```python
from build123d import *

# Parameters (mm, degrees)
SKETCH1_W           = 82.55
SKETCH1_H           = 44.45
BOSS_EXTRUDE1_DEPTH = 6.35
SKETCH2_W           = 5.588
SKETCH2_H           = 18.288
BOSS_EXTRUDE2_DEPTH = 6.35
SKETCH5_W           = 18.288
SKETCH5_H           = 5.588
BOSS_EXTRUDE3_DEPTH = 6.35
SKETCH3_W           = 5.588
SKETCH3_H           = 18.288
CUT_EXTRUDE1_DEPTH  = 97.739994025
SKETCH6_R           = 1.524
CUT_EXTRUDE2_DEPTH  = 97.739994025


with BuildPart() as part:
    # Sketch1 → Boss-Extrude1 (new body)
    with BuildSketch(Plane.XY):
        with Locations((41.275, 22.225)):
            Rectangle(SKETCH1_W, SKETCH1_H)
    extrude(amount=BOSS_EXTRUDE1_DEPTH)

    # Sketch2 → Boss-Extrude2 (add)
    with BuildSketch(Plane.XY.offset(6.35)):
        with Locations((-2.794, 22.225)):
            Rectangle(SKETCH2_W, SKETCH2_H)
    extrude(amount=-BOSS_EXTRUDE2_DEPTH)

    # Sketch5 → Boss-Extrude3 (add)
    with BuildSketch(Plane.XY.offset(6.35)):
        with Locations((38.481, 47.244)):
            Rectangle(SKETCH5_W, SKETCH5_H)
        with Locations((38.481, -2.794)):
            Rectangle(SKETCH5_W, SKETCH5_H)
    extrude(amount=-BOSS_EXTRUDE3_DEPTH)

    # Sketch3 → Cut-Extrude1 (cut, through all)
    with BuildSketch(Plane.XY.offset(6.35)):
        with Locations((79.756, 22.225)):
            Rectangle(SKETCH3_W, SKETCH3_H)
    extrude(amount=-CUT_EXTRUDE1_DEPTH, mode=Mode.SUBTRACT)

    # Sketch6 → Cut-Extrude2 (cut, through all)
    with BuildSketch(Plane.XY.offset(6.35)):
        with Locations((-2.794, 22.225)):
            Circle(SKETCH6_R)
        with Locations((38.481, -2.794)):
            Circle(SKETCH6_R)
        Polygon((67.437, 23.8125), (70.612, 23.8125), (70.612, 26.035), (73.787, 26.035), (73.787, 23.8125), (76.962, 23.8125), (76.962, 20.6375), (73.787, 20.6375), (73.787, 18.415), (70.612, 18.415), (70.612, 20.6375), (67.437, 20.6375), align=None)
    extrude(amount=-CUT_EXTRUDE2_DEPTH, mode=Mode.SUBTRACT)


solid = part.part
```
Design review of the part built by this model. Coordinates are the model's own, in mm. A direction names the side the tool comes from. Coordinates: 2 decimals unless noted, no trailing zeros. Order: outer loops, then holes, each group sorted by start corner. A loop starts at its lowest first (then second) coordinate and runs counter-clockwise, first axis right, second up. Notation, with made-up numbers: M -31,36 L -27,36 A22 ccw -27,47 Z; hole C -3.5,-28.5 d10. An arc over 180 degrees is marked long. Answer as a JSON object with one key per item and string values. Group by question number.
1) Tool access review of faces 4 (the flat face through (65, 0, 3)), 5 (the flat face through (70.612, 20, 3)), 6 (the flat face through (-3, 31.369, 3)), 7 (the flat face through (69, 20.638, 3)): name each direction out of +Z, -Z, +X, -X, +Y, -Y from which nothing blocks a thin tool from reaching the whole face with its end or side.
2) Add section C-C, the plane y = 16. Write out the cut boundary in (x, z), then the cut area to 3 significant figures.
3) Wall thickness on L1, parallel to X at y = 24.5, z = 1.75; L2, parallel to Y at x = 13, z = 1.5; L3, parallel to X at y = 43, z = 2.75: over which ranges is each line inside the solid? List them lowest first.
4) Add section B-B, the plane z = 4.25. Count the separate pieces of the cut face and the enclosed holes in it, then the cut area to 3 significant figures.
5) Add section A-A, the plane x = 68.5. Write out the cut boundary in (y, z), then the cut area to 3 significant figures.
6) Add section D-D, the plane x = 55.5. Write out the cut boundary in (y, z), then the cut area to 3 significant figures.
7) For pin 1 (1.7 mm diameter, centred on y = -3.5, z = 3, fed in from -X); pin 2 (1 mm diameter, centred on x = 75.5, z = 2, fed in from +Y); pin 3 (3.5 mm diameter, centred on x = 75.5, z = 3, fed in from -Y), all flat-tipped, find the tip position at first contact; note any pin that passes through.
8) Mouldability with a two-part tool opening along X and no side actions: class faces 1 (the flat face through (75, 23.812, 3)), 2 (the flat face through (72, 18.415, 3)), 3 (the flat face through (0, 38, 3)) as pulls with the +X half, pulls with the -X half, needs draft (parallel to the pull), parting line crosses it, or undercut.
Computed values:
{
 "1": {"face 4": "+Z, -Z, +X, -Y", "face 5": "+Z, -Z", "face 6": "+Z, -Z, -X, +Y", "face 7": "+Z, -Z, +X"},
 "2": {"outline": "M -5.59,0 L 76.96,0 L 76.96,6.35 L -5.59,6.35 Z", "area": "524 mm^2"},
 "3": {"L1": "x = -5.59 to 70.61, 73.79 to 76.96", "L2": "y = 0 to 44.45", "L3": "x = 0 to 82.55"},
 "4": {"separate pieces": "1", "enclosed holes": "2", "area": "3,810 mm^2"},
 "5": {"outline": "M 0,0 L 20.64,0 L 20.64,6.35 L 0,6.35 Z; M 23.81,0 L 44.45,0 L 44.45,6.35 L 23.81,6.35 Z", "area": "262 mm^2"},
 "6": {"outline": "M 0,0 L 44.45,0 L 44.45,6.35 L 0,6.35 Z", "area": "282 mm^2"},
 "7": {"pin 1": "stops at x = 29.34", "pin 2": "stops at y = 44.45", "pin 3": "stops at y = 0"},
 "8": {"face 1": "needs draft", "face 2": "undercut", "face 3": "pulls with the -X half"}
}
